from build123d import *

# Parameters (mm, degrees)
SKETCH1_W           = 36
SKETCH1_H           = 25
BOSS_EXTRUDE1_DEPTH = 36
SKETCH2_W           = 34.5
SKETCH2_H           = 25
CUT_EXTRUDE1_DEPTH  = 34.5
FILLET1_R           = 1
CUT_EXTRUDE2_DEPTH  = 1.5
CUT_EXTRUDE3_DEPTH  = 1.5


with BuildPart() as part:
    # Sketch1 → Boss-Extrude1 (new body)
    with BuildSketch(Plane(origin=(0, 0, 0), x_dir=(1, 0, 0), z_dir=(0, 1, 0))):
        with Locations((18, 12.5)):
            Rectangle(SKETCH1_W, SKETCH1_H)
    extrude(amount=BOSS_EXTRUDE1_DEPTH)

    # Sketch2 → Cut-Extrude1 (cut)
    with BuildSketch(Plane(origin=(0, 36, 0), x_dir=(1, 0, 0), z_dir=(0, 1, 0))):
        with Locations((18.75, 12.5)):
            Rectangle(SKETCH2_W, SKETCH2_H)
    extrude(amount=-CUT_EXTRUDE1_DEPTH, mode=Mode.SUBTRACT)

    # Fillet1
    fillet1_edges = [part.edges().sort_by_distance(p)[0] for p in [
        (0.75, 36, -25),
        (36, 0.75, -25),
        (36, 0.75, 0),
        (0, 0, -12.5),
        (0.75, 36, 0),
    ]]
    fillet(fillet1_edges, radius=FILLET1_R)

    # Sketch3 → Cut-Extrude2 (cut)
    with BuildSketch(Plane(origin=(0, 1.5, 0), x_dir=(1, 0, 0), z_dir=(0, 1, 0))):
        with BuildLine():
            Line((31, 6.25), (6, 6.25))
            ThreePointArc((6, 6.25), (4.25, 4.5), (6, 2.75))
            Line((6, 2.75), (31, 2.75))
            ThreePointArc((31, 2.75), (32.75, 4.5), (31, 6.25))
        make_face()
        with BuildLine():
            Line((6, 18.75), (31, 18.75))
            ThreePointArc((31, 18.75), (32.75, 20.5), (31, 22.25))
            Line((31, 22.25), (6, 22.25))
            ThreePointArc((6, 22.25), (4.25, 20.5), (6, 18.75))
        make_face()
    extrude(amount=-CUT_EXTRUDE2_DEPTH, mode=Mode.SUBTRACT)

    # Sketch4 → Cut-Extrude3 (cut)
    with BuildSketch(Plane(origin=(1.5, 0, 0), x_dir=(0, 0, -1), z_dir=(1, 0, 0))):
        with BuildLine():
            Line((22.25, 6.5), (22.25, 31.5))
            ThreePointArc((22.25, 31.5), (20.5, 33.25), (18.75, 31.5))
            Line((18.75, 31.5), (18.75, 6.5))
            ThreePointArc((18.75, 6.5), (20.5, 4.75), (22.25, 6.5))
        make_face()
        with BuildLine():
            ThreePointArc((6.25, 31.5), (4.5, 33.25), (2.75, 31.5))
            Line((2.75, 31.5), (2.75, 6.5))
            ThreePointArc((2.75, 6.5), (4.5, 4.75), (6.25, 6.5))
            Line((6.25, 6.5), (6.25, 31.5))
        make_face()
    extrude(amount=-CUT_EXTRUDE3_DEPTH, mode=Mode.SUBTRACT)


solid = part.part
Input: part model. Units: mm. Frame: model coordinates. A direction names the side the tool comes from. Coordinates: 2 decimals unless noted, no trailing zeros. Write each loop counter-clockwise with the first axis right and the second up, starting at its lowest first coordinate (ties: lowest second). Pieces come first, ordered by that corner, then holes. Notation, with made-up numbers: M 39.5,37.25 L 44.5,37.25 A20 cw 44.5,61.25 Z; hole C -15.5,-5.75 d4. An arc over 180 degrees is marked long. Answer as a JSON object with one key per item and string values. Group by question number.
(1) Ray query, line 1 along X through (y, z) = (8.5, -12). Return the intervals inside material, ascending. Write a range as [from, to].
(2) Section D-D on z = -14.25. Output: boundary loops of the cut face in (x, y).
(3) Mould query, pull axis X, two halves, no side actions, for faces 1 (the face through (1, 36, -13)), 2 (the face through (35.699, 0.76, -24.715)), 3 (the face through (19, 1, -6.25)). Classes: pulls with the +X half, pulls with the -X half, needs draft (parallel to the pull), parting line crosses it, or undercut.
(4) Section B-B on y = 16.5. Output: boundary loops of the cut face in (x, z).
(5) Section A-A on z = -20.5. Output: boundary loops of the cut face in (x, y), plus the area to 3 significant figures.
(6) Contact query for flat-ended pins moving along their axis: P1, Ø12.5, axis at y = 19.5, z = -17.5, coming from the +X side; P2, Ø1, axis at x = 16.5, z = -3.5, coming from the -Y side. Output: stop coordinate, or through.
(7) Set-up query: faces 4 (the face through (4.25, 0.76, -4.54)), 5 (the face through (19, 1.5, -13)), 6 (the face through (0.76, 4.75, -20.46)). Return all of +Z, -Z, +X, -X, +Y, -Y with unobstructed straight access to the full face (end or side cutting, diameter ignored); none if empty.
Result set:
{
 "1": {"line 1": "x = [0, 1.5]"},
 "2": {"outline": "M 0,1 A1 ccw 1,0 L 36,0 L 36,1.5 L 1.5,1.5 L 1.5,36 L 0,36 Z"},
 "3": {"face 1": "needs draft", "face 2": "pulls with the +X half", "face 3": "undercut"},
 "4": {"outline": "M 0,-25 L 1.5,-25 L 1.5,-22.25 L 0,-22.25 Z; M 0,-18.75 L 1.5,-18.75 L 1.5,-6.25 L 0,-6.25 Z; M 0,-2.75 L 1.5,-2.75 L 1.5,0 L 0,0 Z"},
 "5": {"outline": "M 0,1 A1 ccw 1,0 L 4.25,0 L 4.25,1.5 L 1.5,1.5 L 1.5,4.75 L 0,4.75 Z; M 0,33.25 L 1.5,33.25 L 1.5,36 L 0,36 Z; M 32.75,0 L 36,0 L 36,1.5 L 32.75,1.5 Z", "area": "20.0 mm2"},
 "6": {"P1": "stops at x = 1.5", "P2": "passes through"},
 "7": {"face 4": "+Y, -Y", "face 5": "+Z, -Z, +X, +Y", "face 6": "+X, -X"}
}
